For this review, take the finished solid that the model builds, in its own axes (mm). A direction names the side the tool comes from. Round coordinates to 2 decimals unless told otherwise and drop trailing zeros. Order: outer loops, then holes, each group sorted by start corner. A loop starts at its lowest first (then second) coordinate and runs counter-clockwise, first axis right, second up. Notation, with made-up numbers: (4.5, 78) - (47.5, 78) arc R22 cw to (47.5, 97) - close; hole circle Ø11 at (-18.5, 9.5). An arc over 180 degrees is marked (long way). One line per item, written item: value.
```python
from build123d import *

# Parameters (mm, degrees)
BOSS_EXTRUDE1_DEPTH  = 20
CUT_EXTRUDE1_START   = -2.5
SKETCH2_R            = 12
SKETCH2_R_2          = 4
CUT_EXTRUDE1_DEPTH   = 15
FILLET1_R            = 2
FILLET1_OF_MIRROR1_R = 2


with BuildPart() as part:
    # Sketch1 → Boss-Extrude1 (new body)
    with BuildSketch(Plane(origin=(0, 0, 0), x_dir=(0, 0, -1), z_dir=(1, 0, 0))):
        with BuildLine():
            Line((0, 0), (-40, 0))
            ThreePointArc((-40, 0), (-62.908712115, -5), (-40, -10))
            Line((-40, -10), (0, -10))
            Line((0, -10), (0, 0))
        make_face()
    boss_extrude1 = extrude(amount=BOSS_EXTRUDE1_DEPTH)

    # Sketch2 → Cut-Extrude1 (cut)
    with BuildSketch(Plane(origin=(20, 0, 0), x_dir=(0, 0, -1), z_dir=(1, 0, 0)).offset(CUT_EXTRUDE1_START)):
        with Locations((-50.908712115, -5)):
            Circle(SKETCH2_R)
        with Locations((-50.908712115, -5)):
            Circle(SKETCH2_R_2, mode=Mode.SUBTRACT)
    cut_extrude1 = extrude(amount=-CUT_EXTRUDE1_DEPTH, mode=Mode.SUBTRACT)

    # Fillet1
    fillet1_edges = [part.edges().sort_by_distance(p)[0] for p in [
        (0, -5, 62.908712115),
        (20, -5, 62.908712115),
        (10, -10, 40),
        (10, 0, 40),
    ]]
    fillet(fillet1_edges, radius=FILLET1_R)

    # Mirror1: Boss-Extrude1, Cut-Extrude1 across plane
    add(boss_extrude1.mirror(Plane(origin=(20, -10, 0), x_dir=(1, 0, 0), z_dir=(0, 0, 1))))
    add(cut_extrude1.mirror(Plane(origin=(20, -10, 0), x_dir=(1, 0, 0), z_dir=(0, 0, 1))), mode=Mode.SUBTRACT)

    # Fillet1 of Mirror1
    fillet1_of_mirror1_edges = [part.edges().sort_by_distance(p)[0] for p in [
        (0, -5, -62.908712115),
        (20, -5, -62.908712115),
        (10, -10, -40),
        (10, 0, -40),
    ]]
    fillet(fillet1_of_mirror1_edges, radius=FILLET1_OF_MIRROR1_R)


solid = part.part
```
Item 1: Machinability: for faces 4 (the cylindrical face through (10.1, -5.04, 38.91)), 5 (the cylindrical face through (17.7, -4.5, -62.9)), which of the approach directions +Z, -Z, +X, -X, +Y, -Y give a long, thin tool a straight path to every point of the face, cutting with its end or side? Answer none if there is none.
Returned:
face 4: none
face 5: +X, -X
Item 2: The part is to be moulded in two halves that separate along Z. For faces 1 (the cylindrical face through (17.7, -4.5, 62.9)), 2 (the flat face through (10, 0, 1)), 3 (the flat face through (0, -5, -1)), say which applies: +Z half, -Z half, draft (parallel to the pull), parting line (faces both ways), or undercut.
Returned:
face 1: undercut
face 2: undercut
face 3: draft
Item 3: Take a section at B-B (z = -27). Write out the cut boundary in (x, y), plus the area to 3 significant figures.
Returned:
outline: (0, -10) - (20, -10) - (20, 0) - (0, 0) - close
area: 200 mm^2
Item 4: For P1, Ø3, axis at x = 6, y = -4.5, coming from the +Z side; P2, Ø8, axis at x = 16.5, y = -13.5, coming from the +Z side; P3, Ø8, axis at x = 15.5, z = -38.5, coming from the -Y side, all flat-tipped, find the tip position at first contact; note any pin that passes through.
Returned:
P1: z = 54.91
P2: z = 61.98
P3: y = -13
Item 5: Take a section at A-A (x = 10.5). Write out the cut boundary in (y, z).
Returned:
outline: (-10, -37.23) arc R2 ccw to (-7.57, -39.19) arc R12 cw to (-2.43, -39.19) arc R2 ccw to (0, -37.23) - (0, 37.23) arc R2 ccw to (-2.43, 39.19) arc R12 cw to (-7.57, 39.19) arc R2 ccw to (-10, 37.23) - close; circle Ø8 at (-5, -50.91); circle Ø8 at (-5, 50.91)
Item 6: Wall thickness on line 1 (Z direction, x = 12.25, y = -7.25); line 2 (X direction, y = -7, z = 58); line 3 (Z direction, x = 5.5, y = -6.5): over which ranges is each line inside the solid? List them lowest first.
Returned:
line 1: -54.22 to -47.6, -39.12 to 39.12, 47.6 to 54.22
line 2: 0 to 2.5, 17.5 to 20
line 3: -54.62 to -47.2, -39 to 39, 47.2 to 54.62
